The model under review builds one solid part; all positions refer to its coordinate system, in mm. A direction names the side the tool comes from. Coordinates: 2 decimals unless noted, no trailing zeros. Order: outer loops, then holes, each group sorted by start corner. A loop starts at its lowest first (then second) coordinate and runs counter-clockwise, first axis right, second up. Notation, with made-up numbers: M -24.75,74 L 12.25,74 A16 cw 12.25,79 Z; hole C 64,13.5 d7. An arc over 180 degrees is marked long. Answer as CSV lines item,"result". Start each with the question number.
Q1. Consider section A-A on x = 19.5. Write out the cut boundary in (y, z).
Q2. Consider section D-D on x = -4. Write out the cut boundary in (y, z), and give its area (3 significant figures).
Q3. Machinability: for faces 1 (the face through (19.486, -0.123, 0.906)), 2 (the face through (-3, 0, -2)), 3 (the face through (-29.5, -2, -50)), 4 (the face through (-25.094, -27.235, -49.765)), which of the approach directions +Z, -Z, +X, -X, +Y, -Y give a long, thin tool a straight path to every point of the face, cutting with its end or side? Answer none if there is none.
Q4. Consider section C-C on y = -14. Write out the cut boundary in (x, z).
Q5. For P1, Ø12.5, axis at y = -2, z = -30, coming from the +X side; P2, Ø10, axis at x = -3.5, y = -0.5, coming from the -Z side, all flat-tipped, find the tip position at first contact; note any pin that passes through.
Q6. Consider section B-B on z = -22. Write out the cut boundary in (x, y), and give its area (3 significant figures).
Q7. Wall thickness on L1, parallel to Y at x = -12.5, z = -40.5; L2, parallel to Y at x = -20, z = -8.5; L3, parallel to X at y = 19.5, z = -50.5: over which ranges is each line inside the solid? List them lowest first. Write a range as [from, to].
from build123d import *

# Parameters (mm, degrees)
F1_DEPTH    = 2
F2_DEPTH    = 103
F3_W        = 50.8
F3_H        = 41.6650772095
F4_DEPTH    = 2
F5_T1_DEPTH = 135.3099275981
F5_T3_DEPTH = 135.2654919008
F6_T1_DEPTH = 41.6650772095


# Not quite as in the source:
# - a fillet or chamfer that OpenCascade refuses, or shapes differently, is made with other operations: its cross-section is extruded or revolved along the edge and cut away or added
# - a feature names something its author has since deleted; it is built from what else it names


with BuildPart() as f1:
    # F0 (on Top) → F1 (new body)
    with BuildSketch(Plane.XY):
        with BuildLine():
            Line((23.2482, -29.5159982), (-19.5, -29.5159982))
            ThreePointArc((-19.5, -29.5159982), (-25.1568542495, -27.1728524495), (-27.5, -21.5159982))
            Line((-27.5, -21.5159982), (-27.5, 20.4840018))
            ThreePointArc((-27.5, 20.4840018), (-25.4213975047, 25.863318819), (-20.2657371023, 28.4472703934))
            Line((-20.2657371023, 28.4472703934), (-18.7638364732, 28.4472703934))
            Line((-18.7638364732, 28.4472703934), (23.2477635268, 28.4774018))
            Line((23.2477635268, 28.4774018), (23.2477635268, 30.4840018))
            Line((23.2477635268, 30.4840018), (-13.8766431592, 30.4840018))
            Line((-13.8766431592, 30.4840018), (-18.7638364732, 30.4840018))
            Line((-18.7638364732, 30.4840018), (-21.4966431592, 30.4840018))
            ThreePointArc((-21.4966431592, 30.4840018), (-27.1487639749, 28.1455855258), (-29.4966319659, 22.4973843711))
            Line((-29.4966319659, 22.4973843711), (-29.5, 20.4840018))
            Line((-29.5, 20.4840018), (-29.5, -21.5159982))
            Line((-29.5, -21.5159982), (-29.5, -23.5159982))
            ThreePointArc((-29.5, -23.5159982), (-27.1568542495, -29.1728524495), (-21.5, -31.5159982))
            Line((-21.5, -31.5159982), (-19.5, -31.5159982))
            Line((-19.5, -31.5159982), (23.2482, -31.5159982))
            Line((23.2482, -31.5159982), (23.2482, -29.5159982))
        make_face()
    extrude(amount=F1_DEPTH)

    # F0 (on Top) → F2 (join)
    with BuildSketch(Plane.XY):
        with BuildLine():
            Line((23.2482, -29.5159982), (-19.5, -29.5159982))
            ThreePointArc((-19.5, -29.5159982), (-25.1568542495, -27.1728524495), (-27.5, -21.5159982))
            Line((-27.5, -21.5159982), (-27.5, 20.4840018))
            ThreePointArc((-27.5, 20.4840018), (-25.4213975047, 25.863318819), (-20.2657371023, 28.4472703934))
            Line((-20.2657371023, 28.4472703934), (-18.7638364732, 28.4472703934))
            Line((-18.7638364732, 28.4472703934), (23.2477635268, 28.4774018))
            Line((23.2477635268, 28.4774018), (23.2477635268, 30.4840018))
            Line((23.2477635268, 30.4840018), (-13.8766431592, 30.4840018))
            Line((-13.8766431592, 30.4840018), (-18.7638364732, 30.4840018))
            Line((-18.7638364732, 30.4840018), (-21.4966431592, 30.4840018))
            ThreePointArc((-21.4966431592, 30.4840018), (-27.1487639749, 28.1455855258), (-29.4966319659, 22.4973843711))
            Line((-29.4966319659, 22.4973843711), (-29.5, 20.4840018))
            Line((-29.5, 20.4840018), (-29.5, -21.5159982))
            Line((-29.5, -21.5159982), (-29.5, -23.5159982))
            ThreePointArc((-29.5, -23.5159982), (-27.1568542495, -29.1728524495), (-21.5, -31.5159982))
            Line((-21.5, -31.5159982), (-19.5, -31.5159982))
            Line((-19.5, -31.5159982), (23.2482, -31.5159982))
            Line((23.2482, -31.5159982), (23.2482, -29.5159982))
        make_face()
    extrude(amount=-F2_DEPTH)

    # F3 (on Top) → F4 (join, symmetric)
    with BuildSketch(Plane.XY):
        with Locations((-4.1, -0.4146657884)):
            Rectangle(F3_W, F3_H)
    extrude(amount=F4_DEPTH, both=True)

    # F5: fillet of radius 10.16 on 2 edges, made by hand

    # F5_s2 → F5_t1 (cut)
    with BuildSketch(Plane.XY.offset(-118.154963799)):
        with BuildLine():
            ThreePointArc((17.1857780072, 30.4840018), (20.3785085, 29.9693152734), (23.2477635268, 28.4774018))
            Line((23.2477635268, 28.4774018), (23.2477635268, 30.4840018))
            Line((23.2477635268, 30.4840018), (17.1857780072, 30.4840018))
        make_face()
    extrude(amount=F5_T1_DEPTH, mode=Mode.SUBTRACT)

    # F5_s4 → F5_t3 (cut)
    with BuildSketch(Plane.XY.offset(-118.1327459504)):
        with BuildLine():
            ThreePointArc((17.1951016198, -31.5159982), (20.3825771099, -31.003049563), (23.2482, -29.5159982))
            Line((23.2482, -29.5159982), (23.2482, -31.5159982))
            Line((23.2482, -31.5159982), (17.1951016198, -31.5159982))
        make_face()
    extrude(amount=F5_T3_DEPTH, mode=Mode.SUBTRACT)

    # F6: fillet of radius 5.08 on 1 edges, made by hand

    # F6_s2 → F6_t1 (cut)
    with BuildSketch(Plane.XZ.offset(-20.4178728163)):
        with BuildLine():
            ThreePointArc((16.3361305416, 2), (19.5236060317, 0.8755530587), (21.3, -2))
            Line((21.3, -2), (21.3, 2))
            Line((21.3, 2), (16.3361305416, 2))
        make_face()
    extrude(amount=F6_T1_DEPTH, mode=Mode.SUBTRACT)


solid = f1.part
Evaluation:
1,outline,"M -31.25,-103 L -29.52,-103 L -29.52,2 L -31.25,2 Z; M -21.25,-2 L 20.42,-2 L 20.42,0.89 L -21.25,0.89 Z; M 28.47,-103 L 30.22,-103 L 30.22,2 L 28.47,2 Z"
2,outline,"M -31.52,-103 L -29.52,-103 L -29.52,2 L -31.52,2 Z; M -21.25,-2 L 20.42,-2 L 20.42,2 L -21.25,2 Z; M 28.46,-103 L 30.48,-103 L 30.48,2 L 28.46,2 Z"
2,area,"589 mm²"
3,face 1,"+Z, +X"
3,face 2,"-Z, +X"
3,face 3,"+Z, -Z, -X, +Y, -Y"
3,face 4,"+Z, -Z, +X"
4,outline,"M -29.5,-103 L -27.5,-103 L -27.5,-2 L 21.3,-2 A5.08 ccw 16.34,2 L -29.5,2 Z"
5,P1,"stops at x = -27.5"
5,P2,"stops at z = -2"
6,outline,"M -29.5,-23.52 A8 ccw -21.5,-31.52 L 17.2,-31.52 A10.16 ccw 23.25,-29.52 L -19.5,-29.52 A8 cw -27.5,-21.52 L -27.5,20.48 A8 cw -20.27,28.45 L -18.76,28.45 L 23.25,28.48 A10.16 ccw 17.19,30.48 L -21.5,30.48 A8 ccw -29.5,22.5 L -29.5,20.48 Z"
6,area,"320 mm²"
7,L1,"y = [-31.52, -29.52], [28.45, 30.48]"
7,L2,"y = [-31.52, -29.5], [28.45, 30.48]"
7,L3,"x = [-29.5, -27.5]"
